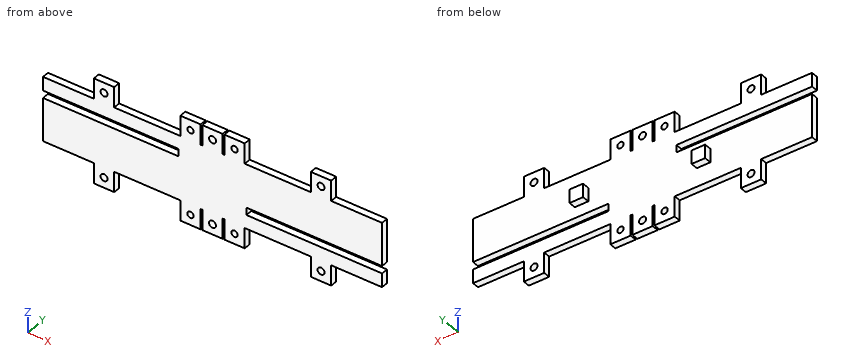
from build123d import *

# Parameters (mm, degrees)
SKETCH1_W           = 160
SKETCH1_H           = 30.4
BOSS_EXTRUDE1_DEPTH = 3.2
SKETCH2_W           = 9.6
SKETCH2_H           = 9.6
SKETCH2_R           = 1.65
BOSS_EXTRUDE2_DEPTH = 3.2
SKETCH3_W           = 64
SKETCH3_H           = 3.5
CUT_EXTRUDE1_DEPTH  = 165.955266663
SKETCH4_W           = 9.6
SKETCH4_H           = 9.6
SKETCH4_R           = 1.5
BOSS_EXTRUDE3_DEPTH = 3.2
SKETCH5_W           = 6.4
SKETCH5_H           = 6.4
BOSS_EXTRUDE4_DEPTH = 3.36


with BuildPart() as part:
    # Sketch1 → Boss-Extrude1 (new body)
    with BuildSketch(Plane(origin=(0, 0, 0), x_dir=(1, 0, 0), z_dir=(0, 1, 0))):
        with Locations((80, -15.2)):
            Rectangle(SKETCH1_W, SKETCH1_H)
    extrude(amount=BOSS_EXTRUDE1_DEPTH)

    # Sketch2 → Boss-Extrude2 (add)
    # profile 1 of 6: a face of its own
    with BuildSketch(Plane(origin=(0, 3.2, 0), x_dir=(1, 0, 0), z_dir=(0, 1, 0))):
        with Locations((28.8, -35.2)):
            Rectangle(SKETCH2_W, SKETCH2_H)
        with Locations(Location((28.8, -35.2, 0), (0, 0, 270))):
            Circle(SKETCH2_R, mode=Mode.SUBTRACT)
    # profile 2 of 6: a face of its own
    with BuildSketch(Plane(origin=(0, 3.2, 0), x_dir=(1, 0, 0), z_dir=(0, 1, 0))):
        with Locations((80, -35.2)):
            Rectangle(SKETCH2_W, SKETCH2_H)
        with Locations(Location((80, -35.2, 0), (0, 0, 270))):
            Circle(SKETCH2_R, mode=Mode.SUBTRACT)
    # profile 3 of 6: a face of its own
    with BuildSketch(Plane(origin=(0, 3.2, 0), x_dir=(1, 0, 0), z_dir=(0, 1, 0))):
        with Locations((131.2, -35.2)):
            Rectangle(SKETCH2_W, SKETCH2_H)
        with Locations(Location((131.2, -35.2, 0), (0, 0, 270))):
            Circle(SKETCH2_R, mode=Mode.SUBTRACT)
    # profile 4 of 6: a face of its own
    with BuildSketch(Plane(origin=(0, 3.2, 0), x_dir=(1, 0, 0), z_dir=(0, 1, 0))):
        with Locations((80, 4.8)):
            Rectangle(SKETCH2_W, SKETCH2_H)
        with Locations(Location((80, 4.8, 0), (0, 0, 270))):
            Circle(SKETCH2_R, mode=Mode.SUBTRACT)
    # profile 5 of 6: a face of its own
    with BuildSketch(Plane(origin=(0, 3.2, 0), x_dir=(1, 0, 0), z_dir=(0, 1, 0))):
        with Locations((131.2, 4.8)):
            Rectangle(SKETCH2_W, SKETCH2_H)
        with Locations(Location((131.2, 4.8, 0), (0, 0, 270))):
            Circle(SKETCH2_R, mode=Mode.SUBTRACT)
    # profile 6 of 6: a face of its own
    with BuildSketch(Plane(origin=(0, 3.2, 0), x_dir=(1, 0, 0), z_dir=(0, 1, 0))):
        with Locations((28.8, 4.8)):
            Rectangle(SKETCH2_W, SKETCH2_H)
        with Locations(Location((28.8, 4.8, 0), (0, 0, 270))):
            Circle(SKETCH2_R, mode=Mode.SUBTRACT)
    extrude(amount=-BOSS_EXTRUDE2_DEPTH)

    # Sketch3 → Cut-Extrude1 (cut, through all)
    with BuildSketch(Plane(origin=(0, 3.2, 0), x_dir=(1, 0, 0), z_dir=(0, 1, 0))):
        with Locations((32, -22.15)):
            Rectangle(SKETCH3_W, SKETCH3_H)
        with Locations((128, -8.25)):
            Rectangle(SKETCH3_W, SKETCH3_H)
    extrude(amount=-CUT_EXTRUDE1_DEPTH, mode=Mode.SUBTRACT)

    # Sketch4 → Boss-Extrude3 (add)
    # profile 1 of 4: a face of its own
    with BuildSketch(Plane(origin=(0, 3.2, 0), x_dir=(1, 0, 0), z_dir=(0, 1, 0))):
        with Locations((69.6, -35.2)):
            Rectangle(SKETCH4_W, SKETCH4_H)
        with Locations(Location((69.6, -35.2, 0), (0, 0, 270))):
            Circle(SKETCH4_R, mode=Mode.SUBTRACT)
    # profile 2 of 4: a face of its own
    with BuildSketch(Plane(origin=(0, 3.2, 0), x_dir=(1, 0, 0), z_dir=(0, 1, 0))):
        with Locations((90.4, -35.2)):
            Rectangle(SKETCH4_W, SKETCH4_H)
        with Locations(Location((90.4, -35.2, 0), (0, 0, 270))):
            Circle(SKETCH4_R, mode=Mode.SUBTRACT)
    # profile 3 of 4: a face of its own
    with BuildSketch(Plane(origin=(0, 3.2, 0), x_dir=(1, 0, 0), z_dir=(0, 1, 0))):
        with Locations((90.4, 4.8)):
            Rectangle(SKETCH4_W, SKETCH4_H)
        with Locations(Location((90.4, 4.8, 0), (0, 0, 90))):
            Circle(SKETCH4_R, mode=Mode.SUBTRACT)
    # profile 4 of 4: a face of its own
    with BuildSketch(Plane(origin=(0, 3.2, 0), x_dir=(1, 0, 0), z_dir=(0, 1, 0))):
        with Locations((69.6, 4.8)):
            Rectangle(SKETCH4_W, SKETCH4_H)
        with Locations(Location((69.6, 4.8, 0), (0, 0, 90))):
            Circle(SKETCH4_R, mode=Mode.SUBTRACT)
    extrude(amount=-BOSS_EXTRUDE3_DEPTH)

    # Sketch5 → Boss-Extrude4 (add)
    with BuildSketch(Plane(origin=(0, 3.2, 0), x_dir=(1, 0, 0), z_dir=(0, 1, 0))):
        with Locations((51.2, -12)):
            Rectangle(SKETCH5_W, SKETCH5_H)
        with Locations((108.8, -18.4)):
            Rectangle(SKETCH5_W, SKETCH5_H)
    extrude(amount=BOSS_EXTRUDE4_DEPTH)


solid = part.part
Model file for the job. Use its own axes, mm. Give positions to 0.01 mm unless a question says otherwise; leave off trailing zeros. Loops run counter-clockwise (first coordinate to the right, second up) from the corner with the lowest first, then second, coordinate; pieces in that order, holes last. Notation, with made-up numbers: (16, 44.25) -> (48, 44.25) arc R28 ccw to (48, 73.25) -> close; hole circle Ø10 at (-28.5, -17.5). An arc over 180 degrees is marked (long way). Use a Markdown table: item, result. Add a question column.
(1) Slice it at C-C on x = 28.8. List the corners of the cut face in (y, z), and give its area (3 significant figures).
(2) Slice it at A-A on y = 5.5. List the corners of the cut face in (x, z).
(3) Slice it at D-D on x = 90.4. List the corners of the cut face in (y, z).
(4) Wall check: line 1 along Z through (x, y) = (131.2, 1.7); line 2 along Z through (x, y) = (69.6, 0.8); line 3 along X through (y, z) = (2.5, 33.5). Give the ranges that are in metal, low to high.
(5) Slice it at B-B on z = 32. List the corners of the cut face in (x, y), and give its area (3 significant figures).
(6) Drop flat-ended pins along their axis: pin 1 Ø2.5 at (y, z) = (4.5, 18.5) entering from -X; pin 2 Ø2.5 at (y, z) = (1, 8) entering from +X; pin 3 Ø3 at (x, z) = (20, 0.5) entering from +Y; pin 4 Ø3 at (x, z) = (80, 35.2) entering from +Y. Give the stop position or say it passes through.
Filled sheet:
| question | item | result |
|---|---|---|
| 1 | outline | (0, -9.6) -> (3.2, -9.6) -> (3.2, -6.45) -> (0, -6.45) -> close; (0, -3.15) -> (3.2, -3.15) -> (3.2, 20.4) -> (0, 20.4) -> close; (0, 23.9) -> (3.2, 23.9) -> (3.2, 33.55) -> (0, 33.55) -> close; (0, 36.85) -> (3.2, 36.85) -> (3.2, 40) -> (0, 40) -> close |
| 1 | area | 126 mm2 |
| 2 | outline | (48, 8.8) -> (54.4, 8.8) -> (54.4, 15.2) -> (48, 15.2) -> close; (105.6, 15.2) -> (112, 15.2) -> (112, 21.6) -> (105.6, 21.6) -> close |
| 3 | outline | (0, -9.6) -> (3.2, -9.6) -> (3.2, -6.3) -> (0, -6.3) -> close; (0, -3.3) -> (3.2, -3.3) -> (3.2, 33.7) -> (0, 33.7) -> close; (0, 36.7) -> (3.2, 36.7) -> (3.2, 40) -> (0, 40) -> close |
| 4 | line 1 | -9.6 to -6.45, -3.15 to 6.5, 10 to 33.55, 36.85 to 40 |
| 4 | line 2 | -9.6 to -6.3, -3.3 to 33.7, 36.7 to 40 |
| 4 | line 3 | 24 to 33.6, 64.8 to 74.4, 75.2 to 84.8, 85.6 to 95.2, 126.4 to 136 |
| 5 | outline | (24, 0) -> (33.6, 0) -> (33.6, 3.2) -> (24, 3.2) -> close; (64.8, 0) -> (74.4, 0) -> (74.4, 3.2) -> (64.8, 3.2) -> close; (75.2, 0) -> (84.8, 0) -> (84.8, 3.2) -> (75.2, 3.2) -> close; (85.6, 0) -> (95.2, 0) -> (95.2, 3.2) -> (85.6, 3.2) -> close; (126.4, 0) -> (136, 0) -> (136, 3.2) -> (126.4, 3.2) -> close |
| 5 | area | 154 mm2 |
| 6 | pin 1 | x = 105.6 |
| 6 | pin 2 | x = 96 |
| 6 | pin 3 | y = 3.2 |
| 6 | pin 4 | through |
